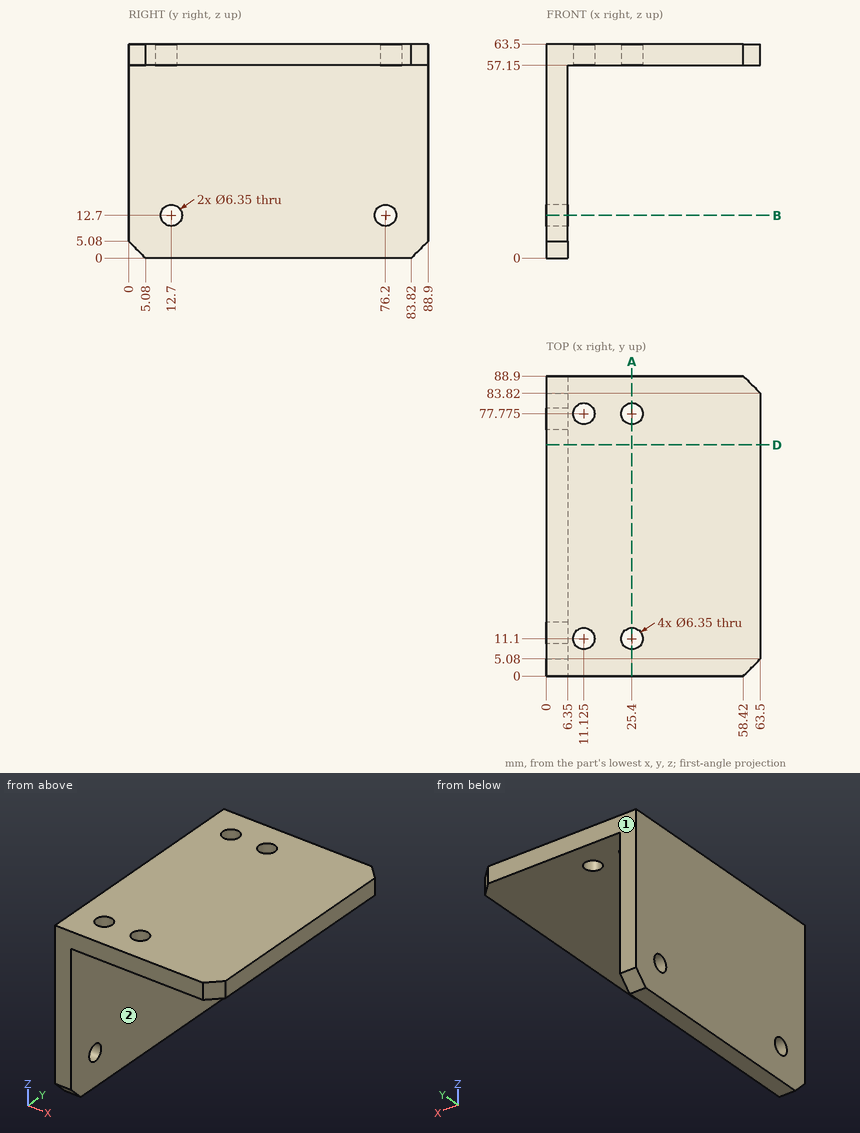
Check sheet for the drawn part. Datum: minimum x, y, z corner. Units: mm. A direction names the side the tool comes from. Round coordinates to 2 decimals unless told otherwise and drop trailing zeros. Write each loop counter-clockwise with the first axis right and the second up, starting at its lowest first coordinate (ties: lowest second). Pieces come first, ordered by that corner, then holes. Notation, with made-up numbers: (5, 52.25) -> (48, 52.25) arc R29 ccw to (48, 81.25) -> close; hole circle Ø2 at (45, -6.75). An arc over 180 degrees is marked (long way). Put each result on its own line as item: value.
(1) Sectioned sample at B-B (z = 12.7). Enter the section's corners in (x, y) (3 decimals), plus the area to 3 significant figures.
Values found:
outline: (0, 0) -> (6.35, 0) -> (6.35, 9.525) -> (0, 9.525) -> close; (0, 15.875) -> (6.35, 15.875) -> (6.35, 73.025) -> (0, 73.025) -> close; (0, 79.375) -> (6.35, 79.375) -> (6.35, 88.9) -> (0, 88.9) -> close
area: 484 mm^2
(2) Tool access check on the marked faces 1 and 2. Record the directions out of +Z, -Z, +X, -X, +Y, -Y that give a thin tool (end or side, any length) a straight path to the whole face; none if there is none.
Values found:
face 1: +Z, -Z, +X, -X, +Y
face 2: -Z, +X, +Y, -Y
(3) Sectioned sample at A-A (x = 25.4). Count the separate pieces of the cut face and the enclosed holes in it, plus the area to 3 significant figures.
Values found:
separate pieces: 3
enclosed holes: 0
area: 484 mm^2
(4) Material ranges on line 1 (Y direction, x = 11.5, z = 57.5); line 2 (X direction, y = 9, z = 26); line 3 (Z direction, x = 57, y = 58), recorded low to high.
Values found:
line 1: y = 0 to 7.95, 14.25 to 74.62, 80.93 to 88.9
line 2: x = 0 to 6.35
line 3: z = 57.15 to 63.5
(5) Sectioned sample at D-D (y = 68.5). Enter the section's corners in (x, z).
Values found:
outline: (0, 0) -> (6.35, 0) -> (6.35, 57.15) -> (63.5, 57.15) -> (63.5, 63.5) -> (0, 63.5) -> close
(6) Go/stop test with flat-tipped pins: pin 1 Ø7.5 at (x, y) = (11.13, 77.77) entering from -Z; pin 2 Ø12 at (y, z) = (49.5, 37.5) entering from +X. Record where each tip stops, or that it passes through.
Values found:
pin 1: stops at z = 57.15
pin 2: stops at x = 6.35
